The model under review builds one solid part; all positions refer to its coordinate system, in mm. Give positions to 0.01 mm unless a question says otherwise; leave off trailing zeros. Write each loop counter-clockwise with the first axis right and the second up, starting at its lowest first coordinate (ties: lowest second). Pieces come first, ordered by that corner, then holes.
from build123d import *

# Parameters (mm, degrees)
SKETCH1_R               = 3
BOSS_EXTRUDE1_DEPTH     = 3
CUT_EXTRUDE1_DEPTH      = 149.690954668
CUT_EXTRUDE1_DEPTH_BACK = 149.690954668
CUT_EXTRUDE2_DEPTH      = 149.690954668
CUT_EXTRUDE2_DEPTH_BACK = 149.690954668
SKETCH4_W               = 10
SKETCH4_H               = 6.1
CUT_EXTRUDE3_DEPTH      = 149.690954668
CUT_EXTRUDE3_DEPTH_BACK = 149.690954668
SKETCH5_W               = 5
SKETCH5_H               = 10
SKETCH6_W               = 3
SKETCH6_H               = 10
SKETCH6_H_2             = 15
CUT_EXTRUDE4_DEPTH      = 149.690954668
CUT_EXTRUDE5_DEPTH      = 149.690954668


with BuildPart() as part:
    # Sketch1 → Boss-Extrude1 (new body)
    with BuildSketch(Plane(origin=(0, 0, 0), x_dir=(0, 0, -1), z_dir=(1, 0, 0))):
        with BuildLine():
            Line((0, 0), (110, 0))
            Line((110, 0), (110, 100))
            Line((110, 100), (85, 100))
            ThreePointArc((85, 100), (24.895923599, 75.104076401), (0, 15))
            Line((0, 15), (0, 0))
        make_face()
        with Locations((50, 80)):
            Circle(SKETCH1_R, mode=Mode.SUBTRACT)
    extrude(amount=BOSS_EXTRUDE1_DEPTH)

    # Sketch2 → Cut-Extrude1 (cut, two sides: drawn at the far end of the back side and taken through both)
    with BuildSketch(Plane(origin=(3, 0, 0), x_dir=(0, 0, -1), z_dir=(1, 0, 0)).offset(-CUT_EXTRUDE1_DEPTH_BACK)):
        with BuildLine():
            Line((110, 0), (75, 0))
            Line((75, 0), (75, 45))
            ThreePointArc((75, 45), (77.928932188, 52.071067812), (85, 55))
            Line((85, 55), (110, 55))
            Line((110, 55), (110, 0))
        make_face()
    extrude(amount=CUT_EXTRUDE1_DEPTH + CUT_EXTRUDE1_DEPTH_BACK, mode=Mode.SUBTRACT)

    # Sketch4 → Cut-Extrude2 (cut, two sides: drawn at the far end of the back side and taken through both)
    with BuildSketch(Plane(origin=(3, 0, 0), x_dir=(0, 0, -1), z_dir=(1, 0, 0)).offset(-CUT_EXTRUDE2_DEPTH_BACK)):
        with Locations((25, 3.05)):
            Rectangle(SKETCH4_W, SKETCH4_H)
        with Locations((5, 3.05)):
            Rectangle(SKETCH4_W, SKETCH4_H)
        with Locations((45, 3.05)):
            Rectangle(SKETCH4_W, SKETCH4_H)
        with Locations((65, 3.05)):
            Rectangle(SKETCH4_W, SKETCH4_H)
    extrude(amount=CUT_EXTRUDE2_DEPTH + CUT_EXTRUDE2_DEPTH_BACK, mode=Mode.SUBTRACT)

    # Sketch5 → Cut-Extrude3 (cut, two sides: drawn at the far end of the back side and taken through both)
    with BuildSketch(Plane.ZY.offset(-CUT_EXTRUDE3_DEPTH_BACK)):
        with Locations((-68.65, 17.6)):
            Rectangle(SKETCH5_W, SKETCH5_H)
        with Locations((-38.65, 17.6)):
            Rectangle(SKETCH5_W, SKETCH5_H)
    extrude(amount=CUT_EXTRUDE3_DEPTH + CUT_EXTRUDE3_DEPTH_BACK, mode=Mode.SUBTRACT)

    # Sketch6 → Cut-Extrude4 (cut, through all)
    with BuildSketch(Plane(origin=(3, 0, 0), x_dir=(0, 0, -1), z_dir=(1, 0, 0))):
        with Locations((106.1, 95)):
            Rectangle(SKETCH6_W, SKETCH6_H)
        with Locations((106.1, 75)):
            Rectangle(SKETCH6_W, SKETCH6_H)
        with Locations((106.1, 52.5)):
            Rectangle(SKETCH6_W, SKETCH6_H_2)
    extrude(amount=-CUT_EXTRUDE4_DEPTH, mode=Mode.SUBTRACT)

    # Sketch7 → Cut-Extrude5 (cut, through all)
    with BuildSketch(Plane(origin=(3, 0, 0), x_dir=(0, 0, -1), z_dir=(1, 0, 0))):
        with BuildLine():
            Line((62.851519915, 50.4125), (59.603924651, 56.0375))
            ThreePointArc((59.603924651, 56.0375), (58.460095264, 57.181329387), (56.897595264, 57.6))
            Line((56.897595264, 57.6), (50.402404736, 57.6))
            ThreePointArc((50.402404736, 57.6), (48.839904736, 57.181329387), (47.696075349, 56.0375))
            Line((47.696075349, 56.0375), (44.448480085, 50.4125))
            ThreePointArc((44.448480085, 50.4125), (44.029809472, 48.85), (44.448480085, 47.2875))
            Line((44.448480085, 47.2875), (47.696075349, 41.6625))
            ThreePointArc((47.696075349, 41.6625), (48.839904736, 40.518670613), (50.402404736, 40.1))
            Line((50.402404736, 40.1), (56.897595264, 40.1))
            ThreePointArc((56.897595264, 40.1), (58.460095264, 40.518670613), (59.603924651, 41.6625))
            Line((59.603924651, 41.6625), (62.851519915, 47.2875))
            ThreePointArc((62.851519915, 47.2875), (63.270190528, 48.85), (62.851519915, 50.4125))
        make_face()
        with BuildLine():
            Line((67.181646934, 44.7875), (63.93405167, 39.1625))
            ThreePointArc((63.93405167, 39.1625), (63.515381057, 37.6), (63.93405167, 36.0375))
            Line((63.93405167, 36.0375), (67.181646934, 30.4125))
            ThreePointArc((67.181646934, 30.4125), (68.06043166, 30.048495448), (68.639479281, 30.803125))
            Line((68.639479281, 30.803125), (68.639479281, 44.396875))
            ThreePointArc((68.639479281, 44.396875), (68.06043166, 45.151504552), (67.181646934, 44.7875))
        make_face()
        with BuildLine():
            Line((62.851519915, 27.9125), (59.603924651, 33.5375))
            ThreePointArc((59.603924651, 33.5375), (58.460095264, 34.681329387), (56.897595264, 35.1))
            Line((56.897595264, 35.1), (50.402404736, 35.1))
            ThreePointArc((50.402404736, 35.1), (48.839904736, 34.681329387), (47.696075349, 33.5375))
            Line((47.696075349, 33.5375), (44.448480085, 27.9125))
            ThreePointArc((44.448480085, 27.9125), (44.029809472, 26.35), (44.448480085, 24.7875))
            Line((44.448480085, 24.7875), (47.696075349, 19.1625))
            ThreePointArc((47.696075349, 19.1625), (48.839904736, 18.018670613), (50.402404736, 17.6))
            Line((50.402404736, 17.6), (56.897595264, 17.6))
            ThreePointArc((56.897595264, 17.6), (58.460095264, 18.018670613), (59.603924651, 19.1625))
            Line((59.603924651, 19.1625), (62.851519915, 24.7875))
            ThreePointArc((62.851519915, 24.7875), (63.270190528, 26.35), (62.851519915, 27.9125))
        make_face()
        with BuildLine():
            Line((43.36594833, 39.1625), (40.118353066, 44.7875))
            ThreePointArc((40.118353066, 44.7875), (38.974523679, 45.931329387), (37.412023679, 46.35))
            Line((37.412023679, 46.35), (30.916833151, 46.35))
            ThreePointArc((30.916833151, 46.35), (29.354333151, 45.931329387), (28.210503764, 44.7875))
            Line((28.210503764, 44.7875), (24.9629085, 39.1625))
            ThreePointArc((24.9629085, 39.1625), (24.544237886, 37.6), (24.9629085, 36.0375))
            Line((24.9629085, 36.0375), (28.210503764, 30.4125))
            ThreePointArc((28.210503764, 30.4125), (29.354333151, 29.268670613), (30.916833151, 28.85))
            Line((30.916833151, 28.85), (37.412023679, 28.85))
            ThreePointArc((37.412023679, 28.85), (38.974523679, 29.268670613), (40.118353066, 30.4125))
            Line((40.118353066, 30.4125), (43.36594833, 36.0375))
            ThreePointArc((43.36594833, 36.0375), (43.784618943, 37.6), (43.36594833, 39.1625))
        make_face()
        with BuildLine():
            Line((23.880376745, 27.9125), (20.632781481, 33.5375))
            ThreePointArc((20.632781481, 33.5375), (19.488952094, 34.681329387), (17.926452094, 35.1))
            Line((17.926452094, 35.1), (11.431261566, 35.1))
            ThreePointArc((11.431261566, 35.1), (9.868761566, 34.681329387), (8.724932179, 33.5375))
            Line((8.724932179, 33.5375), (5.477336915, 27.9125))
            ThreePointArc((5.477336915, 27.9125), (5.058666301, 26.35), (5.477336915, 24.7875))
            Line((5.477336915, 24.7875), (8.724932179, 19.1625))
            ThreePointArc((8.724932179, 19.1625), (9.868761566, 18.018670613), (11.431261566, 17.6))
            Line((11.431261566, 17.6), (17.926452094, 17.6))
            ThreePointArc((17.926452094, 17.6), (19.488952094, 18.018670613), (20.632781481, 19.1625))
            Line((20.632781481, 19.1625), (23.880376745, 24.7875))
            ThreePointArc((23.880376745, 24.7875), (24.299047358, 26.35), (23.880376745, 27.9125))
        make_face()
    extrude(amount=-CUT_EXTRUDE5_DEPTH, mode=Mode.SUBTRACT)


solid = part.part
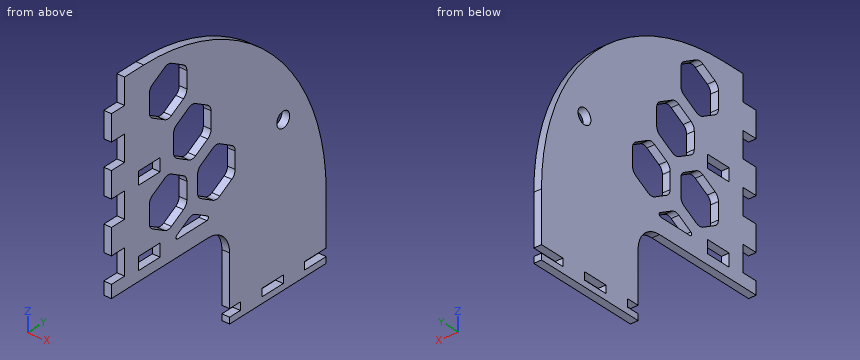
1) Consider section C-C, the plane z = -98. Give the boundary of the cut face in (x, y).
2) Consider section A-A, the plane z = -7.5. Give the boundary of the cut face in (x, y).
3) Consider section D-D, the plane y = 86. Give the boundary of the cut face in (x, z).
4) Insertion check: pin 1 (1.5 mm diameter, centred on x = 2, z = -55, fed in from +Y); pin 2 (5 mm diameter, centred on y = 80, z = -50, fed in from -X); pin 3 (0.9 mm diameter, centred on x = 1.5, z = -6.5, fed in from -Y); pin 4 (0.9 mm diameter, centred on x = 1, y = 30.5, fed in from -Z). Each pin has a flat end and moves straight along its axis. Give the tip position at first contact, or say it passes through.
5) Consider section B-B, the plane x = 2.3. State how many separate pieces and enclosed holes the cut face has, then the cut area to 3 significant figures.
6) To check wall thickness, follow probe 1 along Z at (x, y) = (2.05, 5); probe 2 along Y at (x, z) = (1.85, -54); probe 3 along Z at (x, y) = (2, 57). State the ranges of each line that lie inside material, in increasing order.
Answer block:
1. outline: (0, 55) - (3, 55) - (3, 100) - (0, 100) - close
2. outline: (0, 6.1) - (3, 6.1) - (3, 21.28) - (0, 21.28) - close; (0, 31.42) - (3, 31.42) - (3, 49.91) - (0, 49.91) - close
3. outline: (0, -110) - (3, -110) - (3, -38.27) - (0, -38.27) - close
4. pin 1: stops at y = 94.81
4. pin 2: passes through
4. pin 3: stops at y = 6.1
4. pin 4: stops at z = -75
5. separate pieces: 1
5. enclosed holes: 9
5. area: 6,000 mm2
6. probe 1: z = -75 to -70, -60 to -50, -40 to -30, -20 to -10
6. probe 2: y = 0 to 17.6, 35.1 to 40.1, 57.6 to 94.15
6. probe 3: z = -110 to -107.6, -104.6 to -58.74, -48.56 to -11.1
